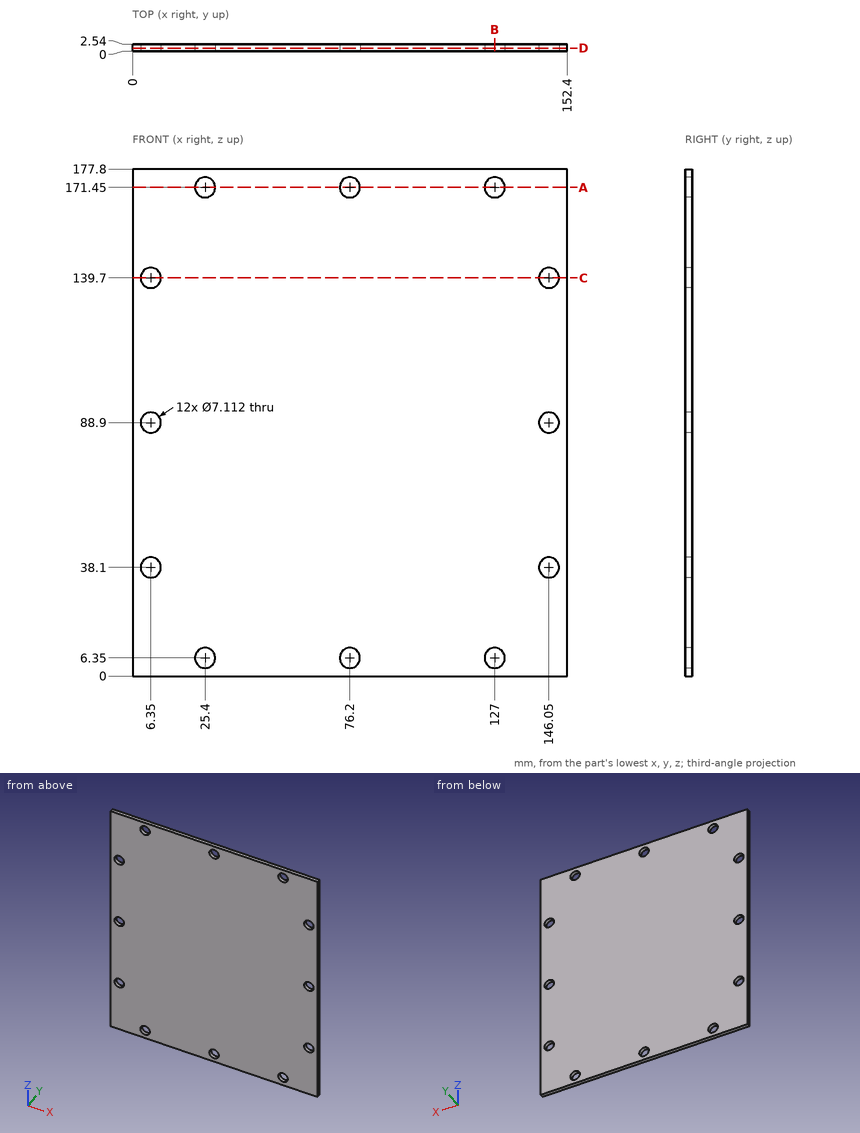
Could you check a few things on this drawing? It's one solid part, dimensions in mm from its lowest x, y, z. Coordinates: 2 decimals unless noted, no trailing zeros. Write each loop counter-clockwise with the first axis right and the second up, starting at its lowest first coordinate (ties: lowest second). Pieces come first, ordered by that corner, then holes. Notation, with made-up numbers: (16.25, -29) - (60.25, -29) arc R13 cw to (60.25, -25) - close; hole circle Ø3 at (42, 3). An arc over 180 degrees is marked (long way). Write item = value, one per line.
1) Suppose I cut it at A-A on z = 171.45. Please give me the cut outline in (x, y).
Result set:
outline = (0, 0) - (21.84, 0) - (21.84, 2.54) - (0, 2.54) - close; (28.96, 0) - (72.64, 0) - (72.64, 2.54) - (28.96, 2.54) - close; (79.76, 0) - (123.44, 0) - (123.44, 2.54) - (79.76, 2.54) - close; (130.56, 0) - (152.4, 0) - (152.4, 2.54) - (130.56, 2.54) - close
2) Suppose I cut it at C-C on z = 139.7. Please give me the cut outline in (x, y).
Result set:
outline = (0, 0) - (2.79, 0) - (2.79, 2.54) - (0, 2.54) - close; (9.91, 0) - (142.49, 0) - (142.49, 2.54) - (9.91, 2.54) - close; (149.61, 0) - (152.4, 0) - (152.4, 2.54) - (149.61, 2.54) - close
3) Will this pin go through, and if not, where does the flat tip stop? pin 1 Ø11.5 at (x, z) = (76.2, 171.45) entering from -Y.
Result set:
pin_1 = 0
4) Please list where these lines run through material, in increasing order: line 1 (X direction, y = 1.55, z = 6.35); line 2 (Z direction, x = 76.2, y = 1.15); line 3 (X direction, y = 1.65, z = 38.1). Write a range as [from, to].
Result set:
line_1 = [0, 21.84], [28.96, 72.64], [79.76, 123.44], [130.56, 152.4]
line_2 = [0, 2.79], [9.91, 167.89], [175.01, 177.8]
line_3 = [0, 2.79], [9.91, 142.49], [149.61, 152.4]
5) Suppose I cut it at B-B on x = 127. Please give me the cut outline in (y, z).
Result set:
outline = (0, 0) - (2.54, 0) - (2.54, 2.79) - (0, 2.79) - close; (0, 9.91) - (2.54, 9.91) - (2.54, 167.89) - (0, 167.89) - close; (0, 175.01) - (2.54, 175.01) - (2.54, 177.8) - (0, 177.8) - close
6) Suppose I cut it at D-D on y = 1.1. State how many separate pieces and enclosed holes the cut face has, plus the area to 3 significant figures.
Result set:
separate_pieces = 1
enclosed_holes = 12
area = 26,600 mm2
